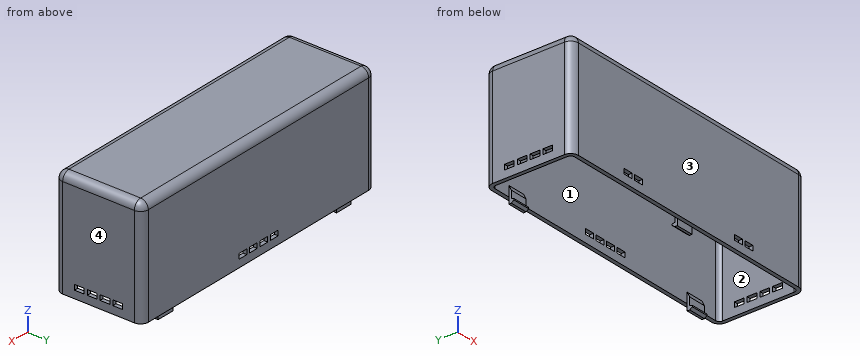
```python
from build123d import *

# Parameters (mm, degrees)
SKETCH1_W             = 111
SKETCH1_H             = 42
BOSS_EXTRUDE1_DEPTH   = 34
FILLET1_R             = 3
SHELL1_T              = -1.5
SKETCH2_W             = 7
SKETCH2_H             = 1
BOSS_EXTRUDE2_DEPTH   = 2.5
BOSS_EXTRUDE2_2_DEPTH = 2.5
BOSS_EXTRUDE2_3_DEPTH = 2.5
SKETCH3_W             = 7
SKETCH3_H             = 1
BOSS_EXTRUDE3_DEPTH   = 4.5
BOSS_EXTRUDE4_DEPTH   = 7
BOSS_EXTRUDE5_DEPTH   = 7
BOSS_EXTRUDE6_DEPTH   = 7
SKETCH7_W             = 7
SKETCH7_H             = 1.5
BOSS_EXTRUDE7_DEPTH   = 1
CUT_EXTRUDE1_REACH    = 149.537
BOSS_EXTRUDE8_DEPTH   = 7
CUT_EXTRUDE3_REACH    = 156.227
SKETCH10_W            = 2
SKETCH10_H            = 3.8
SKETCH11_W            = 3.8
SKETCH11_H            = 2
CUT_EXTRUDE4_DEPTH    = 1.5
SKETCH12_W            = 3.8
SKETCH12_H            = 2
CUT_EXTRUDE5_DEPTH    = 1.5


with BuildPart() as part:
    # Sketch1 → Boss-Extrude1 (new body)
    with BuildSketch(Plane(origin=(0, 0, 0), x_dir=(1, 0, 0), z_dir=(0, 1, 0))):
        with Locations((-152.292726369, -80.532812689)):
            Rectangle(SKETCH1_W, SKETCH1_H)
    extrude(amount=BOSS_EXTRUDE1_DEPTH)

    # Fillet1
    fillet1_edges = [part.edges().sort_by_distance(p)[0] for p in [
        (-96.792726369, 34, 80.532812689),
        (-152.292726369, 34, 101.532812689),
        (-96.792726369, 0, 80.532812689),
        (-207.792726369, 0, 80.532812689),
        (-152.292726369, 0, 101.532812689),
        (-96.792726369, 17, 101.532812689),
        (-207.792726369, 17, 101.532812689),
        (-207.792726369, 34, 80.532812689),
    ]]
    fillet(fillet1_edges, radius=FILLET1_R)

    # Shell1
    shell1_openings = [part.faces().sort_by_distance(p)[0] for p in [
        (-152.292726369, 17, 59.532812689),
    ]]
    offset(amount=SHELL1_T, openings=shell1_openings, kind=Kind.INTERSECTION)



with BuildPart() as body_2:
    # Sketch2 → Boss-Extrude2 (new body)
    with BuildSketch(Plane(origin=(0, 0, 59.532812689), x_dir=(-1, 0, 0), z_dir=(0, 0, -1))):
        with Locations((109.792726369, 32)):
            Rectangle(SKETCH2_W, SKETCH2_H)
    extrude(amount=BOSS_EXTRUDE2_DEPTH)


with BuildPart() as body_3:
    # Sketch2 → Boss-Extrude2 2 (new body)
    with BuildSketch(Plane(origin=(0, 0, 59.532812689), x_dir=(-1, 0, 0), z_dir=(0, 0, -1))):
        with Locations((194.792726369, 32)):
            Rectangle(SKETCH2_W, SKETCH2_H)
    extrude(amount=BOSS_EXTRUDE2_2_DEPTH)


with BuildPart() as body_4:
    # Sketch2 → Boss-Extrude2 3 (new body)
    with BuildSketch(Plane(origin=(0, 0, 59.532812689), x_dir=(-1, 0, 0), z_dir=(0, 0, -1))):
        with Locations((152.292726369, 2)):
            Rectangle(SKETCH2_W, SKETCH2_H)
    extrude(amount=BOSS_EXTRUDE2_3_DEPTH)


with BuildPart() as part_1:
    add(part.part)

    add(body_2.part)  # Boss-Extrude3 merges body 2

    add(body_3.part)  # Boss-Extrude3 merges body 3

    add(body_4.part)  # Boss-Extrude3 merges body 4
    # Sketch3 → Boss-Extrude3 (add)
    with BuildSketch(Plane(origin=(0, 0, 57.032812689), x_dir=(-1, 0, 0), z_dir=(0, 0, -1))):
        with Locations((194.792726369, 32)):
            Rectangle(SKETCH3_W, SKETCH3_H)
        with Locations((109.792726369, 32)):
            Rectangle(SKETCH3_W, SKETCH3_H)
        with Locations((152.292726369, 2)):
            Rectangle(SKETCH3_W, SKETCH3_H)
    extrude(amount=-BOSS_EXTRUDE3_DEPTH)

    # Sketch4 → Boss-Extrude4 (add)
    with BuildSketch(Plane.ZY.offset(113.292726369)):
        Polygon((61.532812689, 31.5), (61.532812689, 32.5), (63.532812689, 32.5), align=None)
    extrude(amount=-BOSS_EXTRUDE4_DEPTH)

    # Sketch5 → Boss-Extrude5 (add)
    with BuildSketch(Plane(origin=(-191.292726369, 0, 0), x_dir=(0, 0, -1), z_dir=(1, 0, 0))):
        Polygon((-61.532812689, 31.5), (-61.532812689, 32.5), (-63.532812689, 32.5), align=None)
    extrude(amount=-BOSS_EXTRUDE5_DEPTH)

    # Sketch6 → Boss-Extrude6 (add)
    with BuildSketch(Plane.ZY.offset(155.792726369)):
        Polygon((61.532812689, 2.5), (61.532812689, 1.5), (63.532812689, 1.5), align=None)
    extrude(amount=-BOSS_EXTRUDE6_DEPTH)

    # Sketch7 → Boss-Extrude7 (add)
    with BuildSketch(Plane.XZ.offset(-31.5)):
        with Locations((-194.792726369, 57.782812689)):
            Rectangle(SKETCH7_W, SKETCH7_H)
        with Locations((-109.792726369, 57.782812689)):
            Rectangle(SKETCH7_W, SKETCH7_H)
    extrude(amount=BOSS_EXTRUDE7_DEPTH)

    # Cut-Extrude1: up to this face of the body (flat: up to its plane)
    cut_extrude1_end = Plane(part_1.part.faces().sort_by_distance((-106.292726369, 31.80952381, 59.378050785))[0])
    # Sketch8 → Cut-Extrude1 (cut, up to the picked face)
    with BuildSketch(Plane.ZY.offset(198.292726369), mode=Mode.PRIVATE) as cut_extrude1_sk1:
        Polygon((57.032812689, 31.5), (57.782812689, 30.5), (57.032812689, 30.5), align=None)
    cut_extrude1_tool1 = split(extrude(cut_extrude1_sk1.sketch, amount=-CUT_EXTRUDE1_REACH, mode=Mode.PRIVATE), bisect_by=cut_extrude1_end, keep=Keep.BOTH, mode=Mode.PRIVATE)
    # Sketch8 → Cut-Extrude1 (cut, up to the picked face)
    with BuildSketch(Plane.ZY.offset(198.292726369), mode=Mode.PRIVATE) as cut_extrude1_sk2:
        Polygon((58.282812689, 30.5), (58.532812689, 31.5), (58.532812689, 30.5), align=None)
    cut_extrude1_tool2 = split(extrude(cut_extrude1_sk2.sketch, amount=-CUT_EXTRUDE1_REACH, mode=Mode.PRIVATE), bisect_by=cut_extrude1_end, keep=Keep.BOTH, mode=Mode.PRIVATE)
    add(cut_extrude1_tool1.solids().sort_by(Axis((-198.292726, 30.833333, 57.282813), (1, 0, 0)))[0], mode=Mode.SUBTRACT)
    add(cut_extrude1_tool2.solids().sort_by(Axis((-198.292726, 30.833333, 58.449479), (1, 0, 0)))[0], mode=Mode.SUBTRACT)

    # Sketch9 → Boss-Extrude8 (add)
    with BuildSketch(Plane.ZY.offset(155.792726369)):
        Polygon((57.032812689, 2.5), (57.782812689, 3.5), (58.282812689, 3.5), (58.532812689, 2.5), align=None)
    extrude(amount=-BOSS_EXTRUDE8_DEPTH)

    # Cut-Extrude3: up to this face of the body (flat: up to its plane)
    cut_extrude3_end = Plane(part_1.part.faces().sort_by_distance((-207.792726369, 17, 79.032812689))[0])
    # Sketch10 → Cut-Extrude3 (cut, up to the picked face)
    with BuildSketch(Plane(origin=(-96.792726369, 0, 0), x_dir=(0, 0, -1), z_dir=(1, 0, 0)), mode=Mode.PRIVATE) as cut_extrude3_sk1:
        with Locations((-63.532812689, 24.5)):
            Rectangle(SKETCH10_W, SKETCH10_H)
    cut_extrude3_tool1 = split(extrude(cut_extrude3_sk1.sketch, amount=-CUT_EXTRUDE3_REACH, mode=Mode.PRIVATE), bisect_by=cut_extrude3_end, keep=Keep.BOTH, mode=Mode.PRIVATE)
    # Sketch10 → Cut-Extrude3 (cut, up to the picked face)
    with BuildSketch(Plane(origin=(-96.792726369, 0, 0), x_dir=(0, 0, -1), z_dir=(1, 0, 0)), mode=Mode.PRIVATE) as cut_extrude3_sk2:
        with Locations((-63.532812689, 19.5)):
            Rectangle(SKETCH10_W, SKETCH10_H)
    cut_extrude3_tool2 = split(extrude(cut_extrude3_sk2.sketch, amount=-CUT_EXTRUDE3_REACH, mode=Mode.PRIVATE), bisect_by=cut_extrude3_end, keep=Keep.BOTH, mode=Mode.PRIVATE)
    # Sketch10 → Cut-Extrude3 (cut, up to the picked face)
    with BuildSketch(Plane(origin=(-96.792726369, 0, 0), x_dir=(0, 0, -1), z_dir=(1, 0, 0)), mode=Mode.PRIVATE) as cut_extrude3_sk3:
        with Locations((-63.532812689, 14.5)):
            Rectangle(SKETCH10_W, SKETCH10_H)
    cut_extrude3_tool3 = split(extrude(cut_extrude3_sk3.sketch, amount=-CUT_EXTRUDE3_REACH, mode=Mode.PRIVATE), bisect_by=cut_extrude3_end, keep=Keep.BOTH, mode=Mode.PRIVATE)
    # Sketch10 → Cut-Extrude3 (cut, up to the picked face)
    with BuildSketch(Plane(origin=(-96.792726369, 0, 0), x_dir=(0, 0, -1), z_dir=(1, 0, 0)), mode=Mode.PRIVATE) as cut_extrude3_sk4:
        with Locations((-63.532812689, 9.5)):
            Rectangle(SKETCH10_W, SKETCH10_H)
    cut_extrude3_tool4 = split(extrude(cut_extrude3_sk4.sketch, amount=-CUT_EXTRUDE3_REACH, mode=Mode.PRIVATE), bisect_by=cut_extrude3_end, keep=Keep.BOTH, mode=Mode.PRIVATE)
    add(cut_extrude3_tool1.solids().sort_by(Axis((-96.792726, 24.5, 63.532813), (-1, 0, 0)))[0], mode=Mode.SUBTRACT)
    add(cut_extrude3_tool2.solids().sort_by(Axis((-96.792726, 19.5, 63.532813), (-1, 0, 0)))[0], mode=Mode.SUBTRACT)
    add(cut_extrude3_tool3.solids().sort_by(Axis((-96.792726, 14.5, 63.532813), (-1, 0, 0)))[0], mode=Mode.SUBTRACT)
    add(cut_extrude3_tool4.solids().sort_by(Axis((-96.792726, 9.5, 63.532813), (-1, 0, 0)))[0], mode=Mode.SUBTRACT)

    # Sketch11 → Cut-Extrude4 (cut)
    with BuildSketch(Plane(origin=(0, 34, 0), x_dir=(1, 0, 0), z_dir=(0, 1, 0))):
        with Locations((-159.792726369, -63.532812689)):
            Rectangle(SKETCH11_W, SKETCH11_H)
        with Locations((-154.792726369, -63.532812689)):
            Rectangle(SKETCH11_W, SKETCH11_H)
        with Locations((-149.792726369, -63.532812689)):
            Rectangle(SKETCH11_W, SKETCH11_H)
        with Locations((-144.792726369, -63.532812689)):
            Rectangle(SKETCH11_W, SKETCH11_H)
    extrude(amount=-CUT_EXTRUDE4_DEPTH, mode=Mode.SUBTRACT)

    # Sketch12 → Cut-Extrude5 (cut)
    with BuildSketch(Plane.XZ):
        with Locations((-123.542726369, 63.532812689)):
            Rectangle(SKETCH12_W, SKETCH12_H)
        with Locations((-128.542726369, 63.532812689)):
            Rectangle(SKETCH12_W, SKETCH12_H)
        with Locations((-176.042726369, 63.532812689)):
            Rectangle(SKETCH12_W, SKETCH12_H)
        with Locations((-181.042726369, 63.532812689)):
            Rectangle(SKETCH12_W, SKETCH12_H)
    extrude(amount=-CUT_EXTRUDE5_DEPTH, mode=Mode.SUBTRACT)


solid = part_1.part
```
Here's how the part is built. I have some questions about the finished solid (model axes, mm). Face numbers are marked on the shaded views. Coordinates: 2 decimals unless noted, no trailing zeros. Loops run counter-clockwise (first coordinate to the right, second up) from the corner with the lowest first, then second, coordinate; pieces in that order, holes last. Notation, with made-up numbers: (35.5, -12) - (62.5, -12) arc R29 ccw to (62.5, 26) - close; hole circle Ø6 at (-27.75, -1.75). An arc over 180 degrees is marked (long way). Return JSON: item names as keys, results as strings. Group by question number.
Item 1: Will these pins go through, and if not, where does the flat tip stop? P1, Ø0.8, axis at x = -97.5, z = 63, coming from the -Y side; P2, Ø0.8, axis at x = -97, y = 9.5, coming from the -Z side; P3, Ø1.6, axis at x = -207, y = 15, coming from the +Z side.
Item 2: We'd pull the mould along X, two halves only. Please class the marked faces 1, 2, 3 and 4: +X half, -X half, draft (parallel to the pull), parting line (faces both ways), or undercut.
Item 3: If we section it at C-C on y = 25: Write out the boundary of the cut face in (x, z), and give its area (3 significant figures).
Item 4: If we section it at B-B on x = -181.5: Write out the boundary of the cut face in (y, z), and give its area (3 significant figures).
Item 5: If we section it at D-D on x = -169.5: Write out the boundary of the cut face in (y, z).
Item 6: I need wall thicknesses on line 1 (X direction, y = 17, z = 70.5); line 2 (Y direction, x = -175.5, z = 72); line 3 (Z direction, x = -153, y = 4). Which ranges of each line are inside material? Lowest first, please. Write a range as from..to.
Item 7: If we section it at A-A on z = 93.5: Write out the boundary of the cut face in (x, y), and give its area (3 significant figures).
Calculated:
{
 "1": {"P1": "stops at y = 0.67", "P2": "stops at z = 59.53", "P3": "stops at z = 101.18"},
 "2": {"face 1": "undercut", "face 2": "undercut", "face 3": "draft", "face 4": "+X half"},
 "3": {"outline": "(-207.79, 59.53) - (-206.29, 59.53) - (-206.29, 62.53) - (-207.79, 62.53) - close; (-207.79, 64.53) - (-206.29, 64.53) - (-206.29, 98.53) arc R1.5 cw to (-204.79, 100.03) - (-99.79, 100.03) arc R1.5 cw to (-98.29, 98.53) - (-98.29, 64.53) - (-96.79, 64.53) - (-96.79, 98.53) arc R3 ccw to (-99.79, 101.53) - (-204.79, 101.53) arc R3 ccw to (-207.79, 98.53) - close; (-98.29, 59.53) - (-96.79, 59.53) - (-96.79, 62.53) - (-98.29, 62.53) - close", "area": "279 mm^2"},
 "4": {"outline": "(0, 59.53) - (1.5, 59.53) - (1.5, 62.53) - (0, 62.53) - close; (0, 64.53) - (1.5, 64.53) - (1.5, 98.53) arc R1.5 cw to (3, 100.03) - (31, 100.03) arc R1.5 cw to (32.5, 98.53) - (32.5, 59.53) - (34, 59.53) - (34, 98.53) arc R3 ccw to (31, 101.53) - (3, 101.53) arc R3 ccw to (0, 98.53) - close", "area": "167 mm^2"},
 "5": {"outline": "(0, 59.53) - (1.5, 59.53) - (1.5, 98.53) arc R1.5 cw to (3, 100.03) - (31, 100.03) arc R1.5 cw to (32.5, 98.53) - (32.5, 59.53) - (34, 59.53) - (34, 98.53) arc R3 ccw to (31, 101.53) - (3, 101.53) arc R3 ccw to (0, 98.53) - close"},
 "6": {"line 1": "x = -207.79..-206.29, -98.29..-96.79", "line 2": "y = 0..1.5, 32.5..34", "line 3": "z = 100.03..101.53"},
 "7": {"outline": "(-207.79, 3) arc R3 ccw to (-204.79, 0) - (-99.79, 0) arc R3 ccw to (-96.79, 3) - (-96.79, 31) arc R3 ccw to (-99.79, 34) - (-204.79, 34) arc R3 ccw to (-207.79, 31) - close; hole (-206.29, 3) arc R1.5 ccw to (-204.79, 1.5) - (-99.79, 1.5) arc R1.5 ccw to (-98.29, 3) - (-98.29, 31) arc R1.5 ccw to (-99.79, 32.5) - (-204.79, 32.5) arc R1.5 ccw to (-206.29, 31) - close", "area": "420 mm^2"}
}
